Check sheet for the modelled part. Datum: model origin and axes. Units: mm. Face numbers are marked on the shaded views. A direction names the side the tool comes from. Round coordinates to 2 decimals unless told otherwise and drop trailing zeros. Loops run counter-clockwise (first coordinate to the right, second up) from the corner with the lowest first, then second, coordinate; pieces in that order, holes last. Notation, with made-up numbers: M -29,61 L -6,61 A21 cw -6,95 Z; hole C -32.75,88 d1. An arc over 180 degrees is marked long. Write item = value, one per line. Start each with the question number.
(1) Cross-section at D-D on y = -36.5. Record the boundary of the cut face in (x, z), plus the area to 3 significant figures.
(2) Cross-section at C-C on z = 12.5. Record the boundary of the cut face in (x, y).
(3) Cross-section at A-A on z = 24.5. Record the boundary of the cut face in (x, y).
(4) Cross-section at B-B on x = 13. Record the boundary of the cut face in (y, z), plus the area to 3 significant figures.
(5) Scan lines: L1, parallel to Y at x = 21.5, z = 32; L2, parallel to Z at x = 9, y = -0.5; L3, parallel to X at y = -39.7, z = 39.5. Record each from-to range of solid material in increasing order. Write a range as from..to.
(6) Set-up check for the marked faces 1 and 2: record each of +Z, -Z, +X, -X, +Y, -Y from which the full face is reachable in a straight line by a thin tool's end or side.
(7) Go/stop test with flat-tipped pins: P1, Ø5, axis at x = 5, z = 35, coming from the +Y side; P2, Ø3, axis at x = 1, y = -3.5, coming from the +Z side. Record where each tip stops, or that it passes through.
Autodesk Inventor part; units mm, degrees
ref_plane "YZ Plane" through (0, 0, 0) normal (1, 0, 0) x (0, 1, 0)
ref_plane "XZ Plane" through (0, 0, 0) normal (0, 1, 0) x (-1, 0, 0)
ref_plane "XY Plane" through (0, 0, 0) normal (0, 0, 1) x (1, 0, 0)
sketch "スケッチ1" plane through (0, 0, 0) normal (0, 0, 1) x (1, 0, 0)
  line L0 (-12.8546, 6.7314) -> (32.1454, 6.7314)
  line L1 (32.1454, 6.7314) -> (32.1454, -38.2686)
  line L2 (32.1454, -38.2686) -> (-12.8546, -38.2686)
  line L3 (-12.8546, -38.2686) -> (-12.8546, 6.7314)
  point P0 (0, 0)
  dimension "d0" = 45
  dimension "d1" = 45
sketch "スケッチ2" plane through (0, 0, 0) normal (0, 0, 1) x (1, 0, 0)
  point P0 (0, 0)
extrude "押し出し1" add sketch "スケッチ1" along normal blind 2
sketch "スケッチ3" plane through (0, 0, 2) normal (0, 0, 1) x (1, 0, 0)
  circle A0 centre (9.6454, -15.7686) radius 4
  line L0 (-12.8546, 6.7314) -> (-12.8546, -38.2686)
  line L1 (32.1454, 6.7314) -> (-12.8546, 6.7314)
  point P0 (0, 0)
  dimension "d4" = 8
  dimension "d5" = 22.5
  dimension "d6" = 45
  dimension "d7" = 22.5
hole "穴1" at (9.6454, -15.7686, 2) direction (0, 0, -1) diameter 8 depth 2
sketch "スケッチ4" plane through (-12.8546, -38.2686, 0) normal (0, -1, 0) x (1, 0, 0)
  line L0 (0, 47) -> (45, 47)
  line L1 (45, 47) -> (45, 0)
  line L2 (45, 0) -> (0, 0)
  line L3 (0, 0) -> (0, 47)
  point P0 (12.8546, 0)
  dimension "d15" = 45
  dimension "d16" = 47
extrude "押し出し2" add sketch "スケッチ4" along normal blind 2
sketch "スケッチ5" plane through (0, 0, 2) normal (0, 0, 1) x (1, 0, 0)
  circle A0 centre (9.6454, -15.7686) radius 7
  line L0 (32.1454, 6.7314) -> (-12.8546, 6.7314)
  line L1 (32.1454, -38.2686) -> (32.1454, 6.7314)
  point P0 (0, 0)
  dimension "d19" = 14
  dimension "d20" = 22.5
  dimension "d21" = 22.5
extrude "押し出し3" cut sketch "スケッチ5" against normal blind 2
sketch "スケッチ6" plane through (-12.8546, -38.2686, 0) normal (0, 1, 0) x (1, 0, 0)
  circle A0 centre (22.5, -9.5) radius 1.5
  circle A1 centre (22.5, -24.5) radius 1.5
  circle A2 centre (22.5, -39.5) radius 1.5
  line L0 (45, -47) -> (45, -2)
  line L1 (0, -47) -> (45, -47)
  point P0 (12.8546, 0)
  dimension "d24" = 3
  dimension "d25" = 3
  dimension "d26" = 3
  dimension "d27" = 22.5
  dimension "d28" = 22.5
  dimension "d29" = 22.5
  dimension "d30" = 7.5
  dimension "d31" = 15
  dimension "d32" = 15
hole "穴2" at (9.6454, -38.2686, 39.5) at (9.6454, -38.2686, 24.5) at (9.6454, -38.2686, 9.5) direction (0, -1, 0) diameter 3 depth 2
equation "\"BendRadius\" = Thickness"
equation "\"BendReliefWidth\" = Thickness"
equation "\"BendReliefDepth\" = 0.5 * Thickness"
equation "\"CornerReliefSize\" = 4 * Thickness"
equation "\"MinimumRemnant\" = 2 * Thickness"
equation "\"TransitionRadius\" = BendRadius"
equation "\"JacobiRadiusSize\" = BendRadius"
equation "\"GapSize\" = Thickness"
properties part number "nhk14" material "アルミニウム 6061"
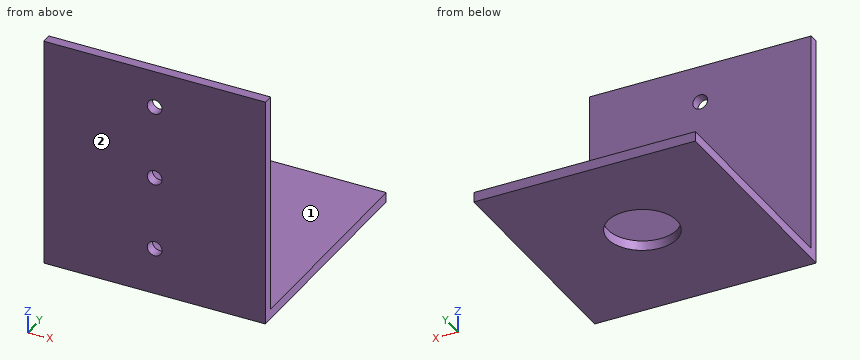
Result:
q1.outline = M -12.85,0 L 32.15,0 L 32.15,2 L -12.85,2 Z
q1.area = 90.0 mm^2
q2.outline = M -12.85,-40.27 L 32.15,-40.27 L 32.15,-38.27 L -12.85,-38.27 Z
q3.outline = M -12.85,-40.27 L 8.15,-40.27 L 8.15,-38.27 L -12.85,-38.27 Z; M 11.15,-40.27 L 32.15,-40.27 L 32.15,-38.27 L 11.15,-38.27 Z
q4.outline = M -40.27,0 L -21.91,0 L -21.91,2 L -38.27,2 L -38.27,47 L -40.27,47 Z; M -9.62,0 L 6.73,0 L 6.73,2 L -9.62,2 Z
q4.area = 159 mm^2
q5.L1 = -40.27..-38.27
q5.L2 = 0..2
q5.L3 = -12.85..8.15, 11.15..32.15
q6.face_1 = +Z, +X, -X, +Y
q6.face_2 = +Z, -Z, +X, -X, -Y
q7.P1 = -38.27
q7.P2 = 2
